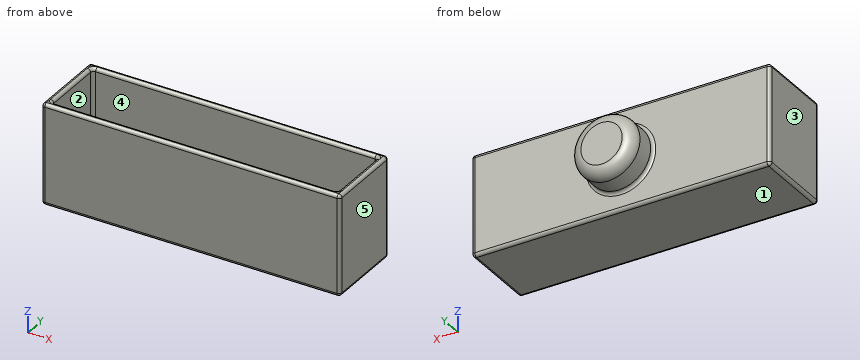
from build123d import *

# Parameters (mm, degrees)
F0_W     = 188
F0_H     = 63.5
F1_DEPTH = 50
F2_W     = 180
F2_H     = 42
F3_DEPTH = 59.5
F4_R     = 20
F5_DEPTH = 20
F6_R     = 7
F7_R     = 1.99999


# Not quite as in the source:
# - a fillet or chamfer is up to 0.001 mm smaller than in the source, because OpenCascade refuses the exact size


with BuildPart() as f1:
    # F0 (on Front) → F1 (new body)
    with BuildSketch(Plane.XZ):
        with Locations((31.2486086041, -31.75)):
            Rectangle(F0_W, F0_H)
    extrude(amount=F1_DEPTH)

    # F2 (on Top) → F3 (cut)
    with BuildSketch(Plane.XY):
        with Locations((31.2486086041, -25)):
            Rectangle(F2_W, F2_H)
    extrude(amount=-F3_DEPTH, mode=Mode.SUBTRACT)

    # F4 (on Front) → F5 (join)
    with BuildSketch(Plane.XZ):
        with Locations((31.2486086041, -31.75)):
            Circle(F4_R)
    extrude(amount=-F5_DEPTH)

    # F6
    f6_edges = [f1.edges().sort_by_distance(p)[0] for p in [
        (11.248609, 20, -31.75),
    ]]
    fillet(f6_edges, radius=F6_R)

    # F7 (radius 2 in the source; OpenCascade refuses exactly that, so slightly less here)
    f7_edges = [f1.edges().sort_by_distance(p)[0] for p in [
        (125.248609, -25, 0),
        (125.248609, -25, -63.5),
        (125.248609, 0, -31.75),
        (125.248609, -50, -31.75),
        (31.248609, 0, 0),
        (-62.751391, -50, -31.75),
        (31.248609, -50, 0),
        (-62.751391, -25, 0),
        (31.248609, -46, 0),
        (121.248609, -25, 0),
        (31.248609, -46, -59.5),
        (31.248609, 0, -63.5),
        (121.248609, -46, -29.75),
        (121.248609, -25, -59.5),
        (31.248609, -4, 0),
        (-58.751391, -25, 0),
        (121.248609, -4, -29.75),
        (31.248609, -4, -59.5),
        (31.248609, -50, -63.5),
        (-58.751391, -46, -29.75),
        (18.248609, 20, -31.75),
        (11.248609, 0, -31.75),
        (11.248609, 13, -31.75),
        (-62.751391, 0, -31.75),
        (-58.751391, -25, -59.5),
        (-58.751391, -4, -29.75),
        (-62.751391, -25, -63.5),
    ]]
    fillet(f7_edges, radius=F7_R)


solid = f1.part
The listing builds one solid part. Answer for the finished solid, in the listing's coordinates (mm). Face numbers are marked on the shaded views. A direction names the side the tool comes from. Coordinates: 2 decimals unless noted, no trailing zeros. Order: outer loops, then holes, each group sorted by start corner. A loop starts at its lowest first (then second) coordinate and runs counter-clockwise, first axis right, second up. Notation, with made-up numbers: M -9.5,28 L -1.5,28 A17 cw -1.5,45 Z; hole C 43,-24 d9. An arc over 180 degrees is marked long. Use CSV: the item, a comma, the result in double quotes.
Q1. Determine the mould class of the marked faces 1, 2 and 3 for opening direction X: pulls with the +X half, pulls with the -X half, needs draft (parallel to the pull), parting line crosses it, or undercut.
Here are the results:
face 1,"needs draft"
face 2,"undercut"
face 3,"pulls with the -X half"
Q2. Straight lines are drawn through the part: L1, parallel to X at y = -39, z = -56; L2, parallel to Y at x = 99.5, z = -43; L3, parallel to Z at x = 79, y = -27.5. For each, find the intervals that lie inside material, in ascending order.
Here are the results:
L1,"-62.75 to -58.75, 121.25 to 125.25"
L2,"-50 to -46, -4 to 0"
L3,"-63.5 to -59.5"
Q3. Section D-D (y = 9) is taken. Determine the outline of the cut face in (x, z), then the cut area to 3 significant figures.
Here are the results:
outline,"C 31.25,-31.75 d40"
area,"1,260 mm2"
Q4. Section C-C (z = -31.75) is taken. Determine the outline of the cut face in (x, y).
Here are the results:
outline,"M -62.75,-48 A2 ccw -60.75,-50 L 123.25,-50 A2 ccw 125.25,-48 L 125.25,-2 A2 ccw 123.25,0 L 53.25,0 A2 cw 51.25,2 L 51.25,13 A7 ccw 44.25,20 L 18.25,20 A7 ccw 11.25,13 L 11.25,2 A2 cw 9.25,0 L -60.75,0 A2 ccw -62.75,-2 Z; hole M -58.75,-44 A2 ccw -56.75,-46 L 119.25,-46 A2 ccw 121.25,-44 L 121.25,-6 A2 ccw 119.25,-4 L -56.75,-4 A2 ccw -58.75,-6 Z"
Q5. Given pin 1 Ø8 at (y, z) = (5, -32) entering from +X; pin 2 Ø8 at (x, z) = (0, -53) entering from +Y; pin 3 Ø11.5 at (x, y) = (67.5, -24.5) entering from +Z, each flat-ended and moving along its own axis, determine where each tip first touches the part or whether it passes through.
Here are the results:
pin 1,"x = 51.52"
pin 2,"y = 0"
pin 3,"z = -59.5"
Q6. A tool of negligible diameter and unlimited length cuts with its end or side. For the marked faces 4 and 5, from which of +Z, -Z, +X, -X, +Y, -Y can it reach the whole face along a straight path? Write none if from no direction.
Here are the results:
face 4,"+Z"
face 5,"+Z, -Z, +X, +Y, -Y"
